```python
from build123d import *

# Parameters (mm, degrees)
F0_W     = 25.4
F0_H     = 6.35
F1_DEPTH = 38.1
F3_DEPTH = 25.4
F4_DEPTH = 12.7
F6_DEPTH = 25.4
F7_DEPTH = 12.7


with BuildPart() as f1:
    # F0 (on Front) → F1 (new body)
    with BuildSketch(Plane.XZ):
        with Locations((12.7, 3.175)):
            Rectangle(F0_W, F0_H)
    extrude(amount=F1_DEPTH)

    # F2 (on Front) → F3 (join)
    with BuildSketch(Plane.XZ):
        Polygon((0, 19.05), (0, 6.35), (15.875, 6.35), (15.875, 12.7), (7.9375, 19.05), align=None)
    extrude(amount=F3_DEPTH)

    # F2 (on Front) → F4 (join)
    with BuildSketch(Plane.XZ):
        Polygon((0, 25.4), (0, 19.05), (7.9375, 19.05), align=None)
    extrude(amount=F4_DEPTH)

    # F5 (on Front) → F6 (join)
    with BuildSketch(Plane.XZ):
        Polygon((25.4, 6.35), (15.875, 12.7), (15.875, 6.35), align=None)
    extrude(amount=F6_DEPTH)

    # F5 (on Front) → F7 (cut)
    with BuildSketch(Plane.XZ):
        Polygon((25.4, 6.35), (15.875, 12.7), (15.875, 6.35), align=None)
    extrude(amount=F7_DEPTH, mode=Mode.SUBTRACT)


solid = f1.part
```
Work out the finished part from the listing and answer in its coordinate system (mm). A direction names the side the tool comes from. Give positions to 0.01 mm unless a question says otherwise; leave off trailing zeros. Order: outer loops, then holes, each group sorted by start corner. A loop starts at its lowest first (then second) coordinate and runs counter-clockwise, first axis right, second up. Notation, with made-up numbers: M -17.75,58.25 L 16.25,58.25 A27 cw 16.25,93.25 Z; hole C -34.5,1 d8. An arc over 180 degrees is marked long. Return JSON: item names as keys, results as strings.
1) A tool of negligible diameter and unlimited length cuts with its end or side. For faces 1 (the flat face through (10, -25.4, 11)), 2 (the flat face through (15.875, -6, 10)), 3 (the flat face through (9.81, -9.7, 17.55)), from which of +Z, -Z, +X, -X, +Y, -Y can it reach the whole face along a straight path? Write none if from no direction.
Resolved:
{"face 1": "+Z, +X, -X, -Y", "face 2": "+Z, +X, +Y", "face 3": "+Z, +X, +Y, -Y"}
2) Section A-A, the plane x = 19.25 is taken. Write down the section's boundary in (y, z).
Resolved:
{"outline": "M -38.1,0 L 0,0 L 0,6.35 L -12.7,6.35 L -12.7,10.45 L -25.4,10.45 L -25.4,6.35 L -38.1,6.35 Z"}
3) Section C-C, the plane z = 11.75 is taken. Write down the section's boundary in (x, y) (3 decimals), plus the area to 3 significant figures.
Resolved:
{"outline": "M 0,-25.4 L 17.3,-25.4 L 17.3,-12.7 L 15.875,-12.7 L 15.875,0 L 0,0 Z", "area": "421 mm^2"}
4) Section B-B, the plane y = -2 is taken. Write down the section's boundary in (x, z) (3 decimals), plus the area to 3 significant figures.
Resolved:
{"outline": "M 0,0 L 25.4,0 L 25.4,6.35 L 15.875,6.35 L 15.875,12.7 L 0,25.4 Z", "area": "363 mm^2"}
5) Section D-D, the plane x = 4.75 is taken. Write down the section's boundary in (y, z), plus the area to 3 significant figures.
Resolved:
{"outline": "M -38.1,0 L 0,0 L 0,21.6 L -12.7,21.6 L -12.7,19.05 L -25.4,19.05 L -25.4,6.35 L -38.1,6.35 Z", "area": "597 mm^2"}
6) Straight lines are drawn through the part: line 1 along Y through (x, z) = (9, 10.25); line 2 along Z through (x, y) = (2.75, -24); line 3 along Y through (x, z) = (7, 19.75). For each, find the intervals that lie inside material, in ascending order. Write a range as [from, to].
Resolved:
{"line 1": "[-25.4, 0]", "line 2": "[0, 19.05]", "line 3": "[-12.7, 0]"}
7) Each of these flat-tipped pins is pushed along its axis until it touches: pin 1 (12 mm diameter, centred on x = 22.5, y = -5.5, fed in from +Z); pin 2 (3 mm diameter, centred on x = 21.5, z = 10.5, fed in from +Y); pin 3 (2.5 mm diameter, centred on x = 5, y = -19, fed in from +Z). Where does it stop, or does it pass through?
Resolved:
{"pin 1": "z = 6.35", "pin 2": "y = -12.7", "pin 3": "z = 19.05"}
